Part print with two shaded views. Sizes in mm from the minimum x, y, z corner. A direction names the side the tool comes from. Coordinates: 2 decimals unless noted, no trailing zeros. Loops run counter-clockwise (first coordinate to the right, second up) from the corner with the lowest first, then second, coordinate; pieces in that order, holes last. Notation, with made-up numbers: (56, 39.5) -> (100, 39.5) arc R35 ccw to (100, 73.5) -> close; hole circle Ø2 at (-10, -31.5). An arc over 180 degrees is marked (long way). Answer as a JSON object with one key per item and string values. Group by question number.
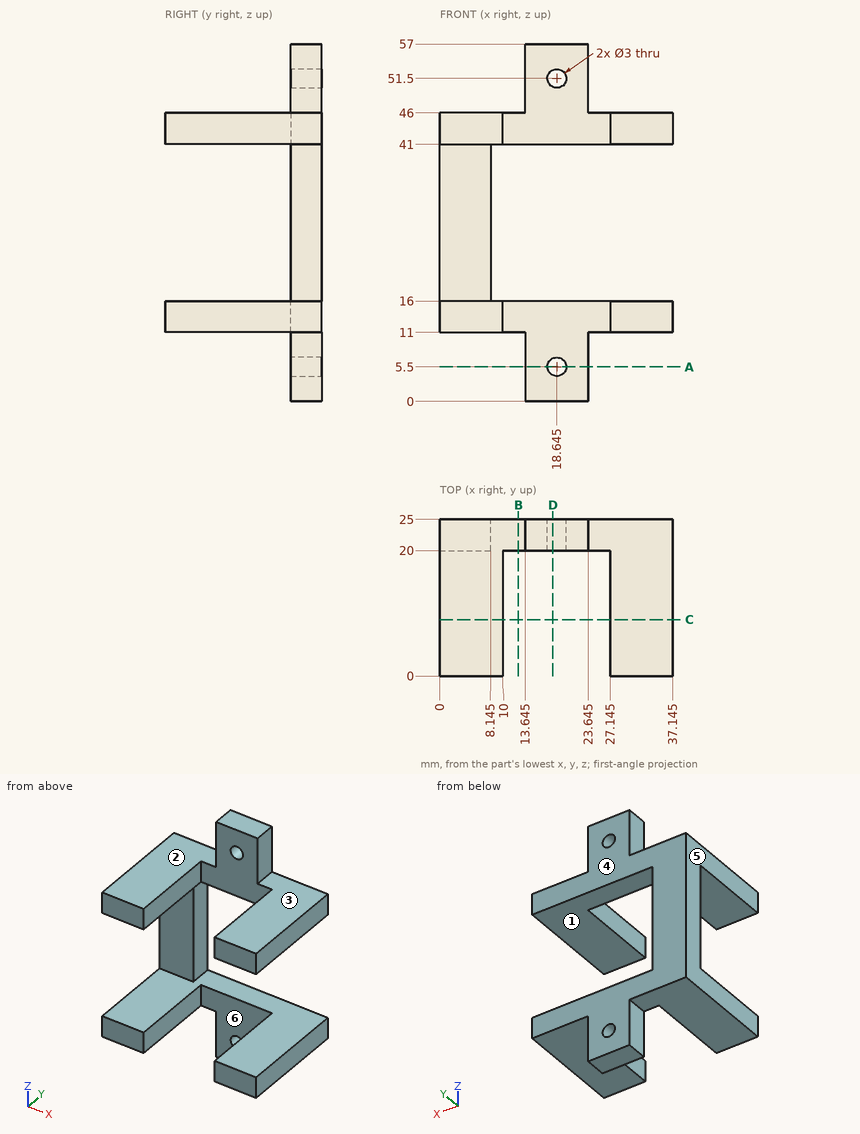
Item 1: Pull direction X, two halves, no side cores. Call the marked faces 4, 5 and 6: +X half, -X half, draft (parallel to the pull), parting line (faces both ways), or undercut.
Item 2: Band-saw the part on D-D, the plane x = 18. List the corners of the cut face in (y, z).
Item 3: Band-saw the part on A-A, the plane z = 5.5. List the corners of the cut face in (x, y) (1 decimal), and give its area (3 significant figures).
Item 4: Band-saw the part on C-C, the plane y = 9. List the corners of the cut face in (x, z) (1 decimal), and give its area (3 significant figures).
Item 5: 3-axis set-ups, long thin cutter, end or side, ignore diameter. For the marked faces 1, 2 and 3: which of +Z, -Z, +X, -X, +Y, -Y reach the whole face in a straight line?
Item 6: Drill centre lines: L1, parallel to X at y = 16, z = 44 (1 decimal); L2, parallel to X at y = 22.05, z = 5.5 (1 decimal); L3, parallel to Z at x = 13, y = 21.5. Where is each one in solid material? Low to high.
Item 7: Flat gauge pins, fed straight in: P1, Ø7.5, axis at x = 11.5, y = 7, coming from the -Z side; P2, Ø2.5, axis at y = 23.5, z = 5, coming from the +X side (3 decimals); P3, Ø11, axis at x = 5.5, y = 8, coming from the +Z side; P4, Ø5, axis at x = 17, z = 17.5, coming from the +Y side. Where does each tip first touch, or does it go through?
Item 8: Band-saw the part on B-B, the plane x = 12.5. List the corners of the cut face in (y, z), and give its area (3 significant figures).
Reply:
{
 "1": {"face 4": "draft", "face 5": "-X half", "face 6": "undercut"},
 "2": {"outline": "(20, 0) -> (25, 0) -> (25, 4.15) -> (20, 4.15) -> close; (20, 6.85) -> (25, 6.85) -> (25, 16) -> (20, 16) -> close; (20, 41) -> (25, 41) -> (25, 50.15) -> (20, 50.15) -> close; (20, 52.85) -> (25, 52.85) -> (25, 57) -> (20, 57) -> close"},
 "3": {"outline": "(13.6, 20) -> (17.1, 20) -> (17.1, 25) -> (13.6, 25) -> close; (20.1, 20) -> (23.6, 20) -> (23.6, 25) -> (20.1, 25) -> close", "area": "35.0 mm²"},
 "4": {"outline": "(0, 11) -> (10, 11) -> (10, 16) -> (0, 16) -> close; (0, 41) -> (10, 41) -> (10, 46) -> (0, 46) -> close; (27.1, 11) -> (37.1, 11) -> (37.1, 16) -> (27.1, 16) -> close; (27.1, 41) -> (37.1, 41) -> (37.1, 46) -> (27.1, 46) -> close", "area": "200 mm²"},
 "5": {"face 1": "+X, -Y", "face 2": "+Z, -X, +Y, -Y", "face 3": "+Z, +X, +Y, -Y"},
 "6": {"L1": "0 to 10, 27.1 to 37.1", "L2": "13.6 to 17.1, 20.1 to 23.6", "L3": "11 to 16, 41 to 46"},
 "7": {"P1": "z = 11", "P2": "x = 23.645", "P3": "z = 46", "P4": "y = 25"},
 "8": {"outline": "(20, 11) -> (25, 11) -> (25, 16) -> (20, 16) -> close; (20, 41) -> (25, 41) -> (25, 46) -> (20, 46) -> close", "area": "50.0 mm²"}
}
